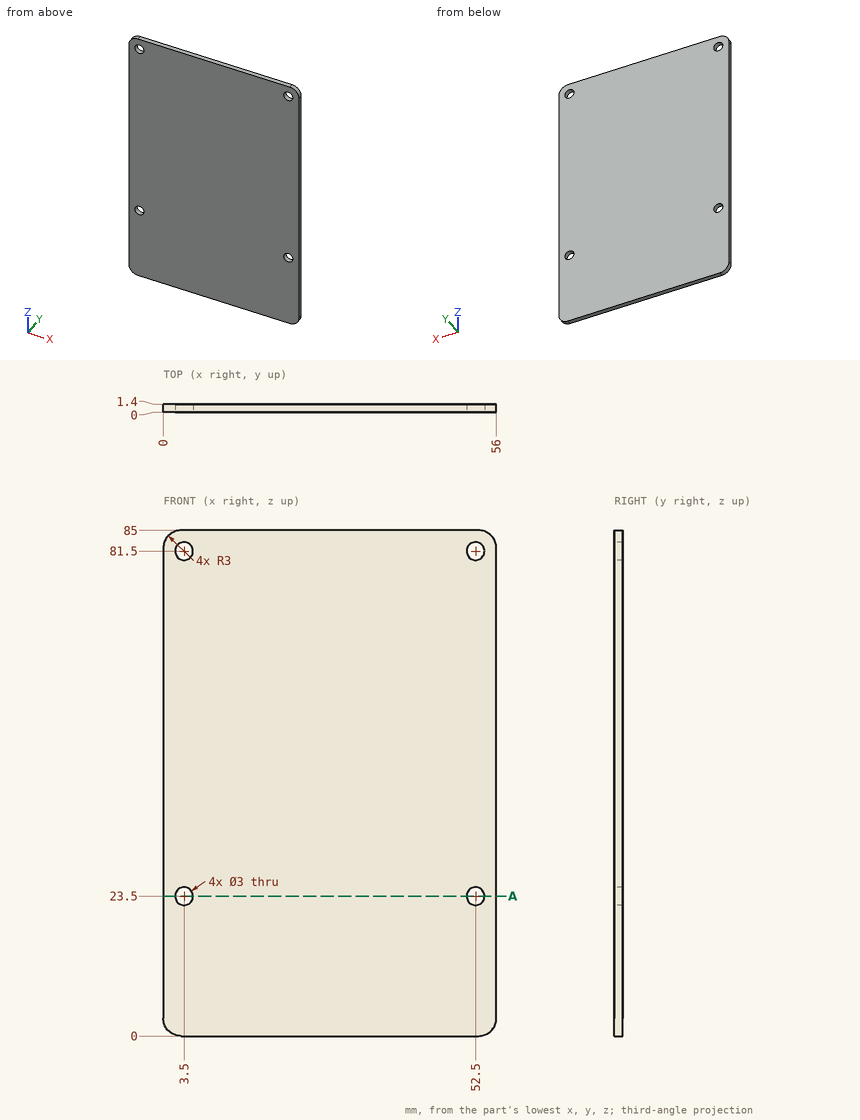
Print and shaded views of the part. All mm, measured from the part's lowest x, y and z. Round coordinates to 2 decimals unless told otherwise and drop trailing zeros. Write each loop counter-clockwise with the first axis right and the second up, starting at its lowest first coordinate (ties: lowest second). Pieces come first, ordered by that corner, then holes. Notation, with made-up numbers: (73, 22) - (106, 22) arc R24 ccw to (106, 53) - close; hole circle Ø8 at (-40, 72). An arc over 180 degrees is marked (long way). Use CSV: the item, a comma, the result in double quotes. Start each with the question number.
Item 1: Drill centre lines: L1, parallel to Z at x = 3.5, y = 0.35; L2, parallel to X at y = 0.7, z = 81.5. Where is each one in solid material? Low to high. Write a range as [from, to].
Item 2: Pin check, flat tips, straight feed: P1, Ø2, axis at x = 7.5, z = 30, coming from the -Y side; P2, Ø2.5, axis at x = 3.5, z = 23.5, coming from the +Y side. Stop position of each tip, or through.
Item 3: Band-saw the part on A-A (z = 23.5). Write the cut outline in (x, y).
Checked values:
1,L1,"z = [0, 22], [25, 80], [83, 85]"
1,L2,"x = [0, 2], [5, 51], [54, 56]"
2,P1,"stops at y = 0"
2,P2,"passes through"
3,outline,"(0, 0) - (2, 0) - (2, 1.4) - (0, 1.4) - close; (5, 0) - (51, 0) - (51, 1.4) - (5, 1.4) - close; (54, 0) - (56, 0) - (56, 1.4) - (54, 1.4) - close"
